from build123d import *

# Parameters (mm, degrees)
SKETCH1_R           = 3.5
BOSS_EXTRUDE1_DEPTH = 10
SKETCH2_R           = 5.9
SKETCH2_R_2         = 3.5
BOSS_EXTRUDE2_DEPTH = 4
SKETCH3_R           = 6.5
BOSS_EXTRUDE3_DEPTH = 1
SKETCH4_R           = 6.5
BOSS_EXTRUDE4_DEPTH = 1
SKETCH5_R           = 5.9
BOSS_EXTRUDE5_DEPTH = 4
BOSS_EXTRUDE6_START = -4.5
SKETCH1_2_R         = 3.5
BOSS_EXTRUDE6_DEPTH = 4.5


with BuildPart() as part:
    # Sketch1 → Boss-Extrude1 (new body)
    with BuildSketch(Plane.XY):
        Circle(SKETCH1_R)
        with BuildLine():
            Line((-1.5, 2), (1.5, 2))
            ThreePointArc((1.5, 2), (0, -2.5), (-1.5, 2))
        make_face(mode=Mode.SUBTRACT)
    extrude(amount=BOSS_EXTRUDE1_DEPTH)

    # Sketch2 → Boss-Extrude2 (add)
    with BuildSketch(Plane(origin=(0, 0, 0), x_dir=(-1, 0, 0), z_dir=(0, 0, -1))):
        with Locations((1, 0)):
            Circle(SKETCH2_R)
        Circle(SKETCH2_R_2, mode=Mode.SUBTRACT)
    extrude(amount=-BOSS_EXTRUDE2_DEPTH)

    # Sketch3 → Boss-Extrude3 (add)
    with BuildSketch(Plane.XY.offset(4)):
        with Locations((-1, 0)):
            Circle(SKETCH3_R)
        with BuildLine():
            Line((1.5, 2), (-1.5, 2))
            ThreePointArc((-1.5, 2), (0, -2.5), (1.5, 2))
        make_face(mode=Mode.SUBTRACT)
    extrude(amount=BOSS_EXTRUDE3_DEPTH)

    # Sketch4 → Boss-Extrude4 (add)
    with BuildSketch(Plane.XY.offset(5)):
        with Locations(Location((1, 0, 0), (0, 0, 261.150116902))):
            Circle(SKETCH4_R)
        with BuildLine():
            Line((1.5, 2), (-1.5, 2))
            ThreePointArc((-1.5, 2), (0, -2.5), (1.5, 2))
        make_face(mode=Mode.SUBTRACT)
    extrude(amount=BOSS_EXTRUDE4_DEPTH)

    # Sketch5 → Boss-Extrude5 (add)
    with BuildSketch(Plane.XY.offset(6)):
        with Locations((1, 0)):
            Circle(SKETCH5_R)
        with BuildLine():
            Line((1.5, 2), (-1.5, 2))
            ThreePointArc((-1.5, 2), (0, -2.5), (1.5, 2))
        make_face(mode=Mode.SUBTRACT)
    extrude(amount=BOSS_EXTRUDE5_DEPTH)

    # Sketch1_2 → Boss-Extrude6 (add)
    with BuildSketch(Plane.XY.offset(BOSS_EXTRUDE6_START)):
        Circle(SKETCH1_2_R)
        with BuildLine():
            Line((-1.5, 2), (1.5, 2))
            ThreePointArc((1.5, 2), (0, -2.5), (-1.5, 2))
        make_face(mode=Mode.SUBTRACT)
    extrude(amount=BOSS_EXTRUDE6_DEPTH)


solid = part.part
Design review of the part built by this model. Coordinates are the model's own, in mm. A direction names the side the tool comes from. Round coordinates to 2 decimals unless told otherwise and drop trailing zeros. Loops run counter-clockwise (first coordinate to the right, second up) from the corner with the lowest first, then second, coordinate; pieces in that order, holes last. Notation, with made-up numbers: (-29, -24.5) - (-13, -24.5) arc R6 ccw to (-13, -15.5) - close; hole circle Ø6 at (24, 5). An arc over 180 degrees is marked (long way). One line per item, written item: value. Start each with the question number.
1) For faces 4 (the cylindrical face through (0.1, -2.5, 2.6)), 5 (the flat face through (6, 0, 5)), 6 (the cylindrical face through (-2.114, 5.705, 5.493)), 7 (the cylindrical face through (-2.409, -6.345, 4.493)), list the 3-axis set-ups (+Z, -Z, +X, -X, +Y, -Y) from which the entire face can be reached by the end or side of a thin tool; tool diameter is ignored.
2) Consider section C-C on z = 4.5. Give the boundary of the cut face in (x, y).
3) Insertion check: pin 1 Ø4 at (y, z) = (3, 1.5) entering from +X; pin 2 Ø2.5 at (x, z) = (0.5, -0.5) entering from -Y; pin 3 Ø2 at (x, y) = (5.5, -4.5) entering from +Z; pin 4 Ø2 at (x, y) = (1.5, 4.5) entering from -Z. Each pin has a flat end and moves straight along its axis. Give the tip position at first contact, or say it passes through.
4) Consider section B-B on y = 0. Give the boundary of the cut face in (x, z).
5) Consider section A-A on x = 0.75. Give the boundary of the cut face in (y, z).
6) To check wall thickness, follow L1, parallel to X at y = 0, z = 5.5; L2, parallel to Z at x = -3.5, y = -4.25; L3, parallel to Y at x = 2.25, z = -3.75. State the ranges of each line that lie inside material, in increasing order. Write a range as from..to.
7) Draft analysis for pull direction X (two halves, no side actions). For faces 1 (the flat face through (0, 2, 3)), 2 (the cylindrical face through (-0.28, -5.76, 7.97)), 3 (the flat face through (-6, 0, 5)), state which applies: +X half, -X half, draft (parallel to the pull), parting line (faces both ways), or undercut.
8) Consider section D-D on x = 6.25. Give the boundary of the cut face in (y, z), then the cut area to 3 significant figures.
Reported:
1. face 4: +Z, -Z
1. face 5: -Z, +X
1. face 6: +Z
1. face 7: -Z
2. outline: circle Ø13 at (-1, 0); hole (-1.5, 2) arc R2.5 ccw (long way) to (1.5, 2) - close
3. pin 1: stops at x = 4.81
3. pin 2: stops at y = -5.89
3. pin 3: stops at z = 10
3. pin 4: stops at z = 0
4. outline: (-7.5, 4) - (-6.9, 4) - (-6.9, 0) - (-3.5, 0) - (-3.5, -4.5) - (-2.5, -4.5) - (-2.5, 10) - (-4.9, 10) - (-4.9, 6) - (-5.5, 6) - (-5.5, 5) - (-7.5, 5) - close; (2.5, -4.5) - (3.5, -4.5) - (3.5, 0) - (4.9, 0) - (4.9, 4) - (5.5, 4) - (5.5, 5) - (7.5, 5) - (7.5, 6) - (6.9, 6) - (6.9, 10) - (2.5, 10) - close
5. outline: (-6.5, 5) - (-6.26, 5) - (-6.26, 4) - (-5.63, 4) - (-5.63, 0) - (-3.42, 0) - (-3.42, -4.5) - (-2.38, -4.5) - (-2.38, 10) - (-5.89, 10) - (-5.89, 6) - (-6.5, 6) - close; (2, -4.5) - (3.42, -4.5) - (3.42, 0) - (5.63, 0) - (5.63, 4) - (6.26, 4) - (6.26, 5) - (6.5, 5) - (6.5, 6) - (5.89, 6) - (5.89, 10) - (2, 10) - close
6. L1: x = -5.5..-2.5, 2.5..7.5
6. L2: z = 0..6
6. L3: y = -2.68..-1.09, 1.09..2.68
7. face 1: undercut
7. face 2: parting line
7. face 3: draft
8. outline: (-3.83, 5) - (3.83, 5) - (3.83, 6) - (2.69, 6) - (2.69, 10) - (-2.69, 10) - (-2.69, 6) - (-3.83, 6) - close
8. area: 29.2 mm^2
